from build123d import *

# Parameters (mm, degrees)
BOSS_EXTRUDE1_DEPTH = 12.7


with BuildPart() as part:
    # Sketch3 → Boss-Extrude1 (new body)
    with BuildSketch(Plane(origin=(0, 0, 0), x_dir=(1, 0, 0), z_dir=(0, 1, 0))):
        with BuildLine():
            Line((-0.79375, 141.285270348), (-0.79375, 125.409988108))
            ThreePointArc((-0.79375, 125.409988108), (-13.1091759, 124.725477203), (-25.297798015, 122.83450888))
            Line((-25.297798015, 122.83450888), (-28.598454788, 138.362878114))
            ThreePointArc((-28.598454788, 138.362878114), (-29.375323016, 138.200029139), (-30.151264104, 138.032818305))
            Line((-30.151264104, 138.032818305), (-26.850607331, 122.504449071))
            ThreePointArc((-26.850607331, 122.504449071), (-38.754593807, 119.27437535), (-50.283710864, 114.890572189))
            Line((-50.283710864, 114.890572189), (-56.74076987, 129.393364168))
            ThreePointArc((-56.74076987, 129.393364168), (-57.466803459, 129.072553847), (-58.191023284, 128.747669747))
            Line((-58.191023284, 128.747669747), (-51.733964278, 114.244877768))
            ThreePointArc((-51.733964278, 114.244877768), (-62.70625, 108.610410952), (-73.071984261, 101.925366188))
            Line((-73.071984261, 101.925366188), (-82.403241037, 114.76873931))
            ThreePointArc((-82.403241037, 114.76873931), (-83.046708833, 114.303988593), (-83.687555516, 113.835630222))
            Line((-83.687555516, 113.835630222), (-74.356298739, 100.9922571))
            ThreePointArc((-74.356298739, 100.9922571), (-83.91734217, 93.199650425), (-92.666661307, 84.505532591))
            Line((-92.666661307, 84.505532591), (-104.464295156, 95.128169822))
            ThreePointArc((-104.464295156, 95.128169822), (-104.99707453, 94.539790546), (-105.526539994, 93.948427412))
            Line((-105.526539994, 93.948427412), (-93.728906144, 83.325790181))
            ThreePointArc((-93.728906144, 83.325790181), (-101.460843807, 73.715617953), (-108.21136059, 63.392401718))
            Line((-108.21136059, 63.392401718), (-121.959758302, 71.330042838))
            ThreePointArc((-121.959758302, 71.330042838), (-122.358564237, 70.64375), (-122.753508302, 69.95522751))
            Line((-122.753508302, 69.95522751), (-109.00511059, 62.01758639))
            ThreePointArc((-109.00511059, 62.01758639), (-114.570019707, 51.00985925), (-119.026704159, 39.508718699))
            Line((-119.026704159, 39.508718699), (-134.124994781, 44.414450702))
            ThreePointArc((-134.124994781, 44.414450702), (-134.372397546, 43.660238593), (-134.61555926, 42.904648482))
            Line((-134.61555926, 42.904648482), (-119.517268638, 37.99891648))
            ThreePointArc((-119.517268638, 37.99891648), (-122.671935977, 26.074724925), (-124.640009603, 13.89831509))
            Line((-124.640009603, 13.89831509), (-140.428325386, 15.557733946))
            ThreePointArc((-140.428325386, 15.557733946), (-140.513512292, 14.768565254), (-140.594264321, 13.978930437))
            Line((-140.594264321, 13.978930437), (-124.805948539, 12.319511581))
            ThreePointArc((-124.805948539, 12.319511581), (-125.4125, 0), (-124.805948539, -12.319511581))
            Line((-124.805948539, -12.319511581), (-140.594264321, -13.978930437))
            ThreePointArc((-140.594264321, -13.978930437), (-140.513512292, -14.768565254), (-140.428325386, -15.557733946))
            Line((-140.428325386, -15.557733946), (-124.640009603, -13.89831509))
            ThreePointArc((-124.640009603, -13.89831509), (-122.671935977, -26.074724925), (-119.517268638, -37.99891648))
            Line((-119.517268638, -37.99891648), (-134.61555926, -42.904648482))
            ThreePointArc((-134.61555926, -42.904648482), (-134.372397546, -43.660238593), (-134.124994781, -44.414450702))
            Line((-134.124994781, -44.414450702), (-119.026704159, -39.508718699))
            ThreePointArc((-119.026704159, -39.508718699), (-114.570019707, -51.00985925), (-109.00511059, -62.01758639))
            Line((-109.00511059, -62.01758639), (-122.753508302, -69.95522751))
            ThreePointArc((-122.753508302, -69.95522751), (-122.358564237, -70.64375), (-121.959758302, -71.330042838))
            Line((-121.959758302, -71.330042838), (-108.21136059, -63.392401718))
            ThreePointArc((-108.21136059, -63.392401718), (-101.460843807, -73.715617953), (-93.728906144, -83.325790181))
            Line((-93.728906144, -83.325790181), (-105.526539994, -93.948427412))
            ThreePointArc((-105.526539994, -93.948427412), (-104.99707453, -94.539790546), (-104.464295156, -95.128169822))
            Line((-104.464295156, -95.128169822), (-92.666661307, -84.505532591))
            ThreePointArc((-92.666661307, -84.505532591), (-83.91734217, -93.199650425), (-74.356298739, -100.9922571))
            Line((-74.356298739, -100.9922571), (-83.687555516, -113.835630222))
            ThreePointArc((-83.687555516, -113.835630222), (-83.046708833, -114.303988593), (-82.403241037, -114.76873931))
            Line((-82.403241037, -114.76873931), (-73.071984261, -101.925366188))
            ThreePointArc((-73.071984261, -101.925366188), (-62.70625, -108.610410952), (-51.733964278, -114.244877768))
            Line((-51.733964278, -114.244877768), (-58.191023284, -128.747669747))
            ThreePointArc((-58.191023284, -128.747669747), (-57.466803459, -129.072553847), (-56.74076987, -129.393364168))
            Line((-56.74076987, -129.393364168), (-50.283710864, -114.890572189))
            ThreePointArc((-50.283710864, -114.890572189), (-38.754593807, -119.27437535), (-26.850607331, -122.504449071))
            Line((-26.850607331, -122.504449071), (-30.151264104, -138.032818305))
            ThreePointArc((-30.151264104, -138.032818305), (-29.375323016, -138.200029139), (-28.598454788, -138.362878114))
            Line((-28.598454788, -138.362878114), (-25.297798015, -122.83450888))
            ThreePointArc((-25.297798015, -122.83450888), (-13.1091759, -124.725477203), (-0.79375, -125.409988108))
            Line((-0.79375, -125.409988108), (-0.79375, -141.285270348))
            ThreePointArc((-0.79375, -141.285270348), (0, -141.2875), (0.79375, -141.285270348))
            Line((0.79375, -141.285270348), (0.79375, -125.409988108))
            ThreePointArc((0.79375, -125.409988108), (13.1091759, -124.725477203), (25.297798015, -122.83450888))
            Line((25.297798015, -122.83450888), (28.598454788, -138.362878114))
            ThreePointArc((28.598454788, -138.362878114), (29.375323016, -138.200029139), (30.151264104, -138.032818305))
            Line((30.151264104, -138.032818305), (26.850607331, -122.504449071))
            ThreePointArc((26.850607331, -122.504449071), (38.754593807, -119.27437535), (50.283710864, -114.890572189))
            Line((50.283710864, -114.890572189), (56.74076987, -129.393364168))
            ThreePointArc((56.74076987, -129.393364168), (57.466803459, -129.072553847), (58.191023284, -128.747669747))
            Line((58.191023284, -128.747669747), (51.733964278, -114.244877768))
            ThreePointArc((51.733964278, -114.244877768), (62.70625, -108.610410952), (73.071984261, -101.925366188))
            Line((73.071984261, -101.925366188), (82.403241037, -114.76873931))
            ThreePointArc((82.403241037, -114.76873931), (83.046708833, -114.303988593), (83.687555516, -113.835630222))
            Line((83.687555516, -113.835630222), (74.356298739, -100.9922571))
            ThreePointArc((74.356298739, -100.9922571), (83.91734217, -93.199650425), (92.666661307, -84.505532591))
            Line((92.666661307, -84.505532591), (104.464295156, -95.128169822))
            ThreePointArc((104.464295156, -95.128169822), (104.99707453, -94.539790546), (105.526539994, -93.948427412))
            Line((105.526539994, -93.948427412), (93.728906144, -83.325790181))
            ThreePointArc((93.728906144, -83.325790181), (101.460843807, -73.715617953), (108.21136059, -63.392401718))
            Line((108.21136059, -63.392401718), (121.959758302, -71.330042838))
            ThreePointArc((121.959758302, -71.330042838), (122.358564237, -70.64375), (122.753508302, -69.95522751))
            Line((122.753508302, -69.95522751), (109.00511059, -62.01758639))
            ThreePointArc((109.00511059, -62.01758639), (114.570019707, -51.00985925), (119.026704159, -39.508718699))
            Line((119.026704159, -39.508718699), (134.124994781, -44.414450702))
            ThreePointArc((134.124994781, -44.414450702), (134.372397546, -43.660238593), (134.61555926, -42.904648482))
            Line((134.61555926, -42.904648482), (119.517268638, -37.99891648))
            ThreePointArc((119.517268638, -37.99891648), (122.671935977, -26.074724925), (124.640009603, -13.89831509))
            Line((124.640009603, -13.89831509), (140.428325386, -15.557733946))
            ThreePointArc((140.428325386, -15.557733946), (140.513512292, -14.768565254), (140.594264321, -13.978930437))
            Line((140.594264321, -13.978930437), (124.805948539, -12.319511581))
            ThreePointArc((124.805948539, -12.319511581), (125.4125, 0), (124.805948539, 12.319511581))
            Line((124.805948539, 12.319511581), (140.594264321, 13.978930437))
            ThreePointArc((140.594264321, 13.978930437), (140.513512292, 14.768565254), (140.428325386, 15.557733946))
            Line((140.428325386, 15.557733946), (124.640009603, 13.89831509))
            ThreePointArc((124.640009603, 13.89831509), (122.671935977, 26.074724925), (119.517268638, 37.99891648))
            Line((119.517268638, 37.99891648), (134.61555926, 42.904648482))
            ThreePointArc((134.61555926, 42.904648482), (134.372397546, 43.660238593), (134.124994781, 44.414450702))
            Line((134.124994781, 44.414450702), (119.026704159, 39.508718699))
            ThreePointArc((119.026704159, 39.508718699), (114.570019707, 51.00985925), (109.00511059, 62.01758639))
            Line((109.00511059, 62.01758639), (122.753508302, 69.95522751))
            ThreePointArc((122.753508302, 69.95522751), (122.358564237, 70.64375), (121.959758302, 71.330042838))
            Line((121.959758302, 71.330042838), (108.21136059, 63.392401718))
            ThreePointArc((108.21136059, 63.392401718), (101.460843807, 73.715617953), (93.728906144, 83.325790181))
            Line((93.728906144, 83.325790181), (105.526539994, 93.948427412))
            ThreePointArc((105.526539994, 93.948427412), (104.99707453, 94.539790546), (104.464295156, 95.128169822))
            Line((104.464295156, 95.128169822), (92.666661307, 84.505532591))
            ThreePointArc((92.666661307, 84.505532591), (83.91734217, 93.199650425), (74.356298739, 100.9922571))
            Line((74.356298739, 100.9922571), (83.687555516, 113.835630222))
            ThreePointArc((83.687555516, 113.835630222), (83.046708833, 114.303988593), (82.403241037, 114.76873931))
            Line((82.403241037, 114.76873931), (73.071984261, 101.925366188))
            ThreePointArc((73.071984261, 101.925366188), (62.70625, 108.610410952), (51.733964278, 114.244877768))
            Line((51.733964278, 114.244877768), (58.191023284, 128.747669747))
            ThreePointArc((58.191023284, 128.747669747), (57.466803459, 129.072553847), (56.74076987, 129.393364168))
            Line((56.74076987, 129.393364168), (50.283710864, 114.890572189))
            ThreePointArc((50.283710864, 114.890572189), (38.754593807, 119.27437535), (26.850607331, 122.504449071))
            Line((26.850607331, 122.504449071), (30.151264104, 138.032818305))
            ThreePointArc((30.151264104, 138.032818305), (29.375323016, 138.200029139), (28.598454788, 138.362878114))
            Line((28.598454788, 138.362878114), (25.297798015, 122.83450888))
            ThreePointArc((25.297798015, 122.83450888), (13.1091759, 124.725477203), (0.79375, 125.409988108))
            Line((0.79375, 125.409988108), (0.79375, 141.285270348))
            ThreePointArc((0.79375, 141.285270348), (0, 141.2875), (-0.79375, 141.285270348))
        make_face()
    extrude(amount=BOSS_EXTRUDE1_DEPTH)


solid = part.part
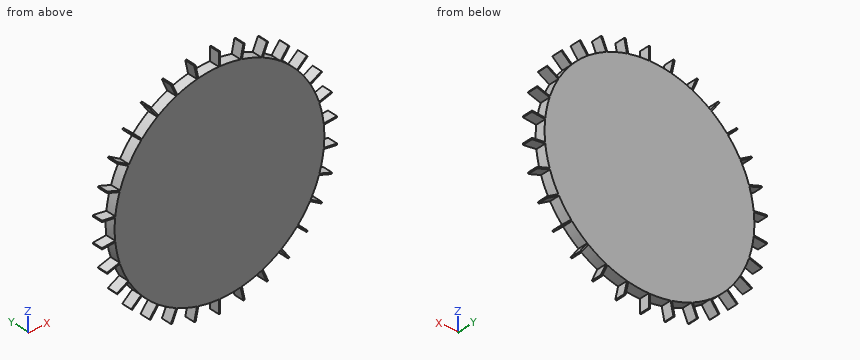
Build history of the part. All positions in model axes, mm. Round coordinates to 2 decimals unless told otherwise and drop trailing zeros. Write each loop counter-clockwise with the first axis right and the second up, starting at its lowest first coordinate (ties: lowest second). Pieces come first, ordered by that corner, then holes. Notation, with made-up numbers: M 2,2 L 56,2 A27 cw 56,39 Z; hole C 20,73.25 d11. An arc over 180 degrees is marked long. Answer in a Markdown table with one row per item.
1. Saw through at C-C (x = -40). List the corners of the cut face in (y, z), and give its area (3 significant figures).
Geometry check:
| item | result |
|---|---|
| outline | M 0,-118.86 L 12.7,-118.86 L 12.7,118.86 L 0,118.86 Z |
| area | 3,020 mm2 |
2. Saw through at B-B (x = 115). List the corners of the cut face in (y, z).
Geometry check:
| item | result |
|---|---|
| outline | M 0,-67.31 L 12.7,-67.31 L 12.7,-65.48 L 0,-65.48 Z; M 0,-50.03 L 12.7,-50.03 L 12.7,50.03 L 0,50.03 Z; M 0,65.48 L 12.7,65.48 L 12.7,67.31 L 0,67.31 Z |
3. Flat gauge pins, fed straight in: P1, Ø5, axis at x = 70, y = 3, coming from the +Z side; P2, Ø4, axis at y = 8.5, z = 134.5, coming from the +X side; P3, Ø1.5, axis at x = -22.5, y = 8, coming from the +Z side. Where does each tip first touch, or does it go through?
Geometry check:
| item | result |
|---|---|
| P1 | z = 105.7 |
| P2 | x = 29.83 |
| P3 | z = 123.51 |
4. Probe L1, parallel to X at y = 10.5, z = 114; L2, parallel to X at y = 5, z = 111; L3, parallel to Z at x = 81.5, y = 2.75. List the from-to ranges inside material, lowest first. Write a range as [from, to].
Geometry check:
| item | result |
|---|---|
| L1 | [-83.46, -81.84], [-52.27, 52.27], [81.84, 83.46] |
| L2 | [-81.63, -79.67], [-58.37, 58.37], [79.67, 81.63] |
| L3 | [-113.53, -110.82], [-95.32, 95.32], [110.82, 113.53] |
5. Saw through at D-D (z = 58). List the corners of the cut face in (x, y), and give its area (3 significant figures).
Geometry check:
| item | result |
|---|---|
| outline | M -111.19,0 L 111.19,0 L 111.19,12.7 L -111.19,12.7 Z |
| area | 2,820 mm2 |
6. Saw through at A-A (z = -107). List the corners of the cut face in (x, y).
Geometry check:
| item | result |
|---|---|
| outline | M -78.72,0 L -76.76,0 L -76.76,12.7 L -78.72,12.7 Z; M -65.42,0 L 65.42,0 L 65.42,12.7 L -65.42,12.7 Z; M 76.76,0 L 78.72,0 L 78.72,12.7 L 76.76,12.7 Z |
